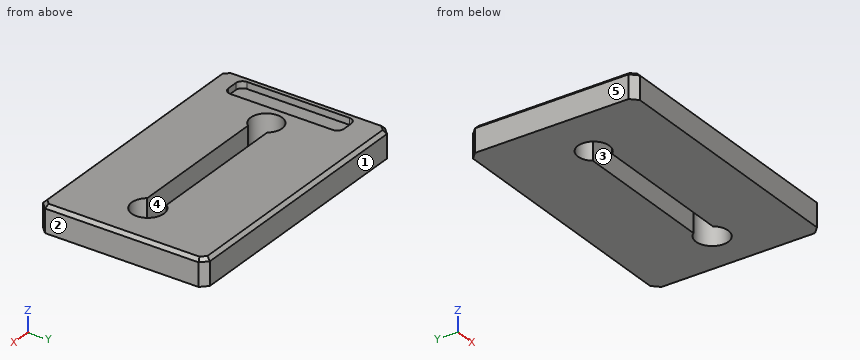
```python
from build123d import *

# Parameters (mm, degrees)
F0_W     = 80
F0_H     = 50
F1_DEPTH = 8
F3_DEPTH = 25.4
F5_DEPTH = 2
F6_SIZE  = 2
F7_SIZE  = 1


with BuildPart() as f1:
    # F0 (on Top) → F1 (new body)
    with BuildSketch(Plane.XY):
        with Locations((-26.7566908151, 1.4298928609)):
            Rectangle(F0_W, F0_H)
    extrude(amount=F1_DEPTH)

    # F2 (on face) → F3 (cut)
    with BuildSketch(Plane.XY.offset(8)):
        with BuildLine():
            ThreePointArc((-3.870154056, -2.8950243141), (4.8331416487, 0), (-3.870154056, 2.8950243141))
            Line((-3.870154056, 2.8950243141), (-47.0229552257, 2.8950243141))
            ThreePointArc((-47.0229552257, 2.8950243141), (-55.4596716368, 0.1073182684), (-47.0969311879, -2.8950243141))
            Line((-47.0969311879, -2.8950243141), (-3.870154056, -2.8950243141))
        make_face()
    extrude(amount=-F3_DEPTH, mode=Mode.SUBTRACT)

    # F4 (on face) → F5 (cut)
    with BuildSketch(Plane.XY.offset(8)):
        with BuildLine():
            ThreePointArc((-57.3456808925, 15.3201337457), (-57.9314673301, 16.734347308), (-59.3456808925, 17.3201337457))
            Line((-59.3456808925, 17.3201337457), (-62.5092031037, 17.3201337457))
            ThreePointArc((-62.5092031037, 17.3201337457), (-63.9234166661, 16.734347308), (-64.5092031037, 15.3201337457))
            Line((-64.5092031037, 15.3201337457), (-64.5092031037, -15.3201337457))
            ThreePointArc((-64.5092031037, -15.3201337457), (-63.9234166661, -16.734347308), (-62.5092031037, -17.3201337457))
            Line((-62.5092031037, -17.3201337457), (-59.3456808925, -17.3201337457))
            ThreePointArc((-59.3456808925, -17.3201337457), (-57.9314673301, -16.734347308), (-57.3456808925, -15.3201337457))
            Line((-57.3456808925, -15.3201337457), (-57.3456808925, 15.3201337457))
        make_face()
    extrude(amount=-F5_DEPTH, mode=Mode.SUBTRACT)

    # F6
    f6_edges = [f1.edges().sort_by_distance(p)[0] for p in [
        (13.243309, 26.429893, 4),
        (13.243309, -23.570107, 4),
        (-66.756691, -23.570107, 4),
        (-66.756691, 26.429893, 4),
    ]]
    chamfer(f6_edges, length=F6_SIZE)

    # F7
    f7_edges = [f1.edges().sort_by_distance(p)[0] for p in [
        (-66.756691, 1.429893, 8),
        (-26.756691, 26.429893, 8),
        (-65.756691, 25.429893, 8),
        (-65.756691, -22.570107, 8),
        (13.243309, 1.429893, 8),
        (12.243309, 25.429893, 8),
        (12.243309, -22.570107, 8),
        (-26.756691, -23.570107, 8),
    ]]
    chamfer(f7_edges, length=F7_SIZE)


solid = f1.part
```
Geometry check sheet. Reference: the model listing, model coordinates, mm. Face numbers are marked on the shaded views. A direction names the side the tool comes from. Round coordinates to 2 decimals unless told otherwise and drop trailing zeros. Loops run counter-clockwise (first coordinate to the right, second up) from the corner with the lowest first, then second, coordinate; pieces in that order, holes last. Notation, with made-up numbers: (-6.75, 10) -> (0.25, 10) arc R23 cw to (0.25, 36) -> close; hole circle Ø1 at (30, -29.75). An arc over 180 degrees is marked (long way). Use a Markdown table: item, result.
(1) Sectioned sample at D-D (x = -39). Enter the section's corners in (y, z).
Calculated:
| item | result |
|---|---|
| outline | (-23.57, 0) -> (-2.9, 0) -> (-2.9, 8) -> (-22.57, 8) -> (-23.57, 7) -> close; (2.9, 0) -> (26.43, 0) -> (26.43, 7) -> (25.43, 8) -> (2.9, 8) -> close |
(2) Go/stop test with a flat-tipped pin: P1, Ø0.6, axis at x = -60.5, z = 7.5, coming from the -Y side. Record where the tip stops, or that it passes through.
Calculated:
| item | result |
|---|---|
| P1 | y = -23.37 |
(3) Scan lines: probe 1 along Y at (x, z) = (-44, 5); probe 2 along Y at (x, z) = (0, 3.5); probe 3 along X at (y, z) = (15, 6.25). Record each from-to range of solid material in increasing order.
Calculated:
| item | result |
|---|---|
| probe 1 | -23.57 to -2.9, 2.9 to 26.43 |
| probe 2 | -23.57 to -4.83, 4.83 to 26.43 |
| probe 3 | -66.76 to -64.51, -57.35 to 13.24 |
(4) Mould release check, pull along X, two halves, no side actions. Record for the marked faces 1, 2 and 3: released by +X, released by -X, zero draft, split by the parting line, or undercut.
Calculated:
| item | result |
|---|---|
| face 1 | zero draft |
| face 2 | released by +X |
| face 3 | undercut |
(5) Set-up check for the marked faces 4 and 5: record each of +Z, -Z, +X, -X, +Y, -Y from which the full face is reachable in a straight line by a thin tool's end or side.
Calculated:
| item | result |
|---|---|
| face 4 | +Z, -Z |
| face 5 | +Z, -Z, -X, +Y, -Y |
(6) Sectioned sample at A-A (x = 0). Enter the section's corners in (y, z).
Calculated:
| item | result |
|---|---|
| outline | (-23.57, 0) -> (-4.83, 0) -> (-4.83, 8) -> (-22.57, 8) -> (-23.57, 7) -> close; (4.83, 0) -> (26.43, 0) -> (26.43, 7) -> (25.43, 8) -> (4.83, 8) -> close |
(7) Sectioned sample at B-B (y = 0). Enter the section's corners in (x, z).
Calculated:
| item | result |
|---|---|
| outline | (-66.76, 0) -> (-55.46, 0) -> (-55.46, 8) -> (-57.35, 8) -> (-57.35, 6) -> (-64.51, 6) -> (-64.51, 8) -> (-65.76, 8) -> (-66.76, 7) -> close; (4.83, 0) -> (13.24, 0) -> (13.24, 7) -> (12.24, 8) -> (4.83, 8) -> close |
(8) Sectioned sample at C-C (z = 4.5). Enter the section's corners in (x, y), then the cut area to 3 significant figures.
Calculated:
| item | result |
|---|---|
| outline | (-66.76, -21.57) -> (-64.76, -23.57) -> (11.24, -23.57) -> (13.24, -21.57) -> (13.24, 24.43) -> (11.24, 26.43) -> (-64.76, 26.43) -> (-66.76, 24.43) -> close; hole (-47.1, -2.9) -> (-3.87, -2.9) arc R4.83 ccw (long way) to (-3.87, 2.9) -> (-47.02, 2.9) arc R4.7 ccw (long way) to start |
| area | 3,610 mm² |
